from build123d import *

# Parameters (mm, degrees)
F1_DEPTH = 152.4


with BuildPart() as f1:
    # F0 (on Front) → F1 (new body)
    with BuildSketch(Plane.XZ):
        Polygon((-76.169543, 76.035284), (-76.169543, 67.358479), (-76.169543, -76.455206), (76.309301, -76.455206), (76.449059, -74.917838), (76.588824, 67.358479), (76.161504, 76.035284), (51.361255, 67.358479), (29.954717, 76.035284), (21.731475, 67.358479), (0, 76.035284), (-19.123683, 67.358479), (-28.913258, 76.035284), (-50.189264, 67.358479), align=None)
        Polygon((3.625234, -71.103098), (-2.087809, -70.939283), (-8.245876, -61.780341), (-6.149467, -52.835658), (0, -50.705924), (6.428989, -52.835658), (8.607126, -59.124887), align=None, mode=Mode.SUBTRACT)
        Polygon((-71.148954, -1.168579), (-48.882278, -1.168579), (-71.148954, -60.398426), align=None, mode=Mode.SUBTRACT)
        with BuildLine():
            Line((-11.182051, -70.944449), (-71.148954, -70.30195))
            Line((-71.148954, -70.30195), (-71.148954, -69.259472))
            Line((-71.148954, -69.259472), (-47.38087, -2.771367))
            Line((-47.38087, -2.771367), (-2.087809, -2.771367))
            Line((-2.087809, -2.771367), (-2.087809, -30.61372))
            Line((-2.087809, -30.61372), (-2.087809, -47.310491))
            ThreePointArc((-2.087809, -47.310491), (-10.455808, -53.241436), (-11.182051, -63.472373))
            Line((-11.182051, -63.472373), (-11.182051, -70.944449))
        make_face(mode=Mode.SUBTRACT)
        with BuildLine():
            Line((1.213909, -2.771367), (50.868321, -2.771367))
            Line((50.868321, -2.771367), (74.797623, -71.865655))
            Line((74.797623, -71.865655), (10.656672, -71.178434))
            Line((10.656672, -71.178434), (10.656672, -64.63617))
            ThreePointArc((10.656672, -64.63617), (10.598486, -53.50252), (1.412784, -47.210906))
            Line((1.412784, -47.210906), (1.412784, -30.61372))
            Line((1.412784, -30.61372), (1.213909, -2.771367))
        make_face(mode=Mode.SUBTRACT)
        Polygon((74.797623, -63.553585), (53.123125, -0.969895), (74.797623, -0.991187), align=None, mode=Mode.SUBTRACT)
        Polygon((-71.148954, 2.174516), (-71.148954, 59.095334), (-49.278473, 2.174516), align=None, mode=Mode.SUBTRACT)
        Polygon((-2.493593, 2.557827), (-47.399332, 2.626492), (-60.058687, 35.574137), (-2.729424, 35.574137), align=None, mode=Mode.SUBTRACT)
        Polygon((-54.496676, 66.376239), (-73.553719, 67.358479), (-73.553719, 72.249986), align=None, mode=Mode.SUBTRACT)
        Polygon((-61.455923, 39.210627), (-71.148954, 64.438023), (-2.939075, 64.925237), (-2.754758, 39.120867), align=None, mode=Mode.SUBTRACT)
        Polygon((-22.386873, 67.358479), (-46.926074, 67.358479), (-30.218534, 73.685788), align=None, mode=Mode.SUBTRACT)
        Polygon((50.849744, 2.47626), (1.725206, 2.551376), (1.489346, 35.571639), (63.597905, 36.015273), align=None, mode=Mode.SUBTRACT)
        Polygon((53.563669, 2.172005), (74.797623, 61.571211), (74.797623, 2.151146), align=None, mode=Mode.SUBTRACT)
        Polygon((1.279462, 64.95537), (74.797623, 65.4805), (65.016477, 39.747379), (1.459519, 39.747379), align=None, mode=Mode.SUBTRACT)
        Polygon((16.510369, 67.358479), (-12.727827, 67.358479), (0, 73.685788), align=None, mode=Mode.SUBTRACT)
        Polygon((44.950325, 67.766275), (26.822057, 67.358479), (30.346299, 73.685788), align=None, mode=Mode.SUBTRACT)
        Polygon((73.713515, 67.766275), (57.104468, 67.766275), (73.681489, 72.249986), align=None, mode=Mode.SUBTRACT)
    extrude(amount=F1_DEPTH)


solid = f1.part
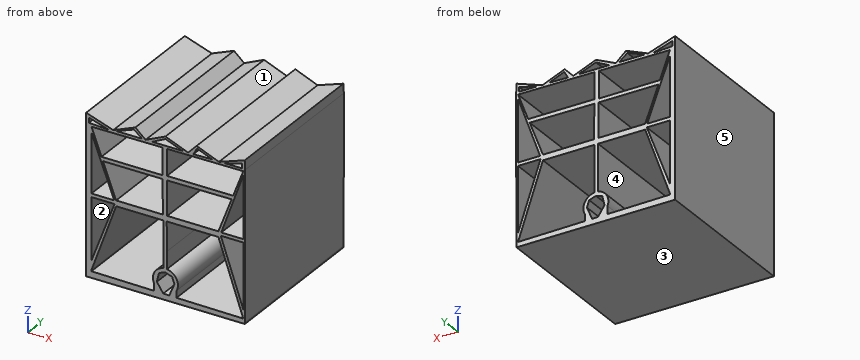
Work out the finished part from the listing and answer in its coordinate system (mm). Face numbers are marked on the shaded views. A direction names the side the tool comes from. Coordinates: 2 decimals unless noted, no trailing zeros. Write each loop counter-clockwise with the first axis right and the second up, starting at its lowest first coordinate (ties: lowest second). Pieces come first, ordered by that corner, then holes.
1. For a pull along Z with two mould halves and no side action, classify the marked faces 1, 2 and 3 as +Z half, -Z half, draft (parallel to the pull), parting line (faces both ways), or undercut.
Results list:
face 1: +Z half
face 2: undercut
face 3: -Z half
2. The part is cut by section A-A, the plane x = -17. Write down the section's boundary in (y, z).
Results list:
outline: (-152.4, -76.46) - (0, -76.46) - (0, -70.88) - (-152.4, -70.88) - close; (-152.4, -2.77) - (0, -2.77) - (0, 2.58) - (-152.4, 2.58) - close; (-152.4, 35.57) - (0, 35.57) - (0, 39.14) - (-152.4, 39.14) - close; (-152.4, 64.82) - (0, 64.82) - (0, 68.32) - (-152.4, 68.32) - close
3. The part is cut by section D-D, the plane y = -127.5. State how many separate pieces and enclosed holes the cut face has, and give its area (3 significant figures).
Results list:
separate pieces: 1
enclosed holes: 16
area: 4,870 mm2
4. Flat-ended cylindrical pins translate along their axes: pin 1 (19.5 mm diameter, centred on x = -38, y = -78.5, fed in from +Z); pin 2 (10 mm diameter, centred on y = -122.5, z = -37.5, fed in from +X); pin 3 (5 mm diameter, centred on x = -58.5, y = -51, fed in from +Z). Find the tip coordinate at first contact, or state that the pin passes through.
Results list:
pin 1: stops at z = 76.04
pin 2: stops at x = 76.49
pin 3: stops at z = 70.97
5. For the marked faces 4 and 5, determine the directions among +Z, -Z, +X, -X, +Y, -Y from which every point of the face is accessible in a straight line to the end or side of a thin tool.
Results list:
face 4: +Y, -Y
face 5: +Z, -Z, -X, +Y, -Y
6. Consider line 1 along X through (y, z) = (-125, -7.5); line 2 along Z through (x, y) = (16, -34.5); line 3 along Z through (x, y) = (30.5, -49). Determine where each line is inside the solid, lowest interval first.
Results list:
line 1: x = -76.17 to -71.15, -51.26 to -49.07, -2.09 to 1.25, 52.51 to 55.38, 74.8 to 76.52
line 2: z = -76.46 to -71.24, -2.77 to 2.53, 35.68 to 39.75, 65.06 to 67.36, 67.55 to 69.65
line 3: z = -76.46 to -71.39, -2.77 to 2.51, 35.78 to 39.75, 65.16 to 67.44, 73.62 to 75.81
7. The part is cut by section C-C, the plane x = 34. Write down the section's boundary in (y, z).
Results list:
outline: (-152.4, -76.46) - (0, -76.46) - (0, -71.43) - (-152.4, -71.43) - close; (-152.4, -2.77) - (0, -2.77) - (0, 2.5) - (-152.4, 2.5) - close; (-152.4, 35.8) - (0, 35.8) - (0, 39.75) - (-152.4, 39.75) - close; (-152.4, 65.19) - (0, 65.19) - (0, 67.52) - (-152.4, 67.52) - close; (-152.4, 72.2) - (0, 72.2) - (0, 74.4) - (-152.4, 74.4) - close
8. The part is cut by section B-B, the plane z = 22. Write down the section's boundary in (x, y).
Results list:
outline: (-76.17, -152.4) - (-71.15, -152.4) - (-71.15, 0) - (-76.17, 0) - close; (-56.9, -152.4) - (-54.84, -152.4) - (-54.84, 0) - (-56.9, 0) - close; (-2.63, -152.4) - (1.59, -152.4) - (1.59, 0) - (-2.63, 0) - close; (58.27, -152.4) - (60.65, -152.4) - (60.65, 0) - (58.27, 0) - close; (74.8, -152.4) - (76.54, -152.4) - (76.54, 0) - (74.8, 0) - close
